Autodesk Fusion 360 part; units mm, degrees
sketch "Sketch1" plane through (0, 0, 0) normal (0, 1, 0) x (1, 0, 0)
  circle A0 centre (0, 0) radius 45
  circle A1 centre (0, 0) radius 2.95
  line L0 (-1.9653, 2.2) -> (1.9653, 2.2)
  circle A2 centre (0, 0) radius 35
  circle A3 centre (0, 0) radius 10
  line L1 (-3.25, 34.8488) -> (-3.25, 9.4571)
  line L2 (3.25, 34.8488) -> (3.25, 9.4571)
  line L3 (-34.1475, 7.6779) -> (-9.9986, -0.1685)
  line L4 (-32.1389, 13.8598) -> (-7.99, 6.0134)
  line L5 (-17.8543, -30.1036) -> (-2.9295, -9.5613)
  line L6 (-23.1129, -26.283) -> (-8.1881, -5.7407)
  line L7 (23.1129, -26.283) -> (8.1881, -5.7407)
  line L8 (17.8543, -30.1036) -> (2.9295, -9.5613)
  line L9 (32.1389, 13.8598) -> (7.99, 6.0134)
  line L10 (34.1475, 7.6779) -> (9.9986, -0.1685)
  line L11 (-0.5, -2.9073) -> (-0.5, -9.9875)
  line L12 (0.5, -2.9073) -> (0.5, -9.9875)
  circle A4 centre (0, 0) radius 42
  dimension "d1" = 90
  dimension "d2" = 5.9
  dimension "d3" = 2.2
  dimension "d4" = 70
  dimension "d5" = 20
  dimension "d6" = 6.5
  dimension "d8" = 360
  dimension "d9" = 1
  dimension "d10" = 84
  dimension "d25" = 25.3916
  dimension "d26" = 20
extrude "Extrude1" add sketch "Sketch1" along normal mid plane 5 contours A0
extrude "Extrude2" add sketch "Sketch1" along normal mid plane 8 contours A4
extrude "Extrude6" add sketch "Sketch1" along normal mid plane 8 contours A1 L0 | A1 A3 L11 L12 | A2 A3 L7 L8 | A2 A3 L5 L6 | A2 A3 L9 L10 | A2 A3 L3 L4 | A2 A3 L1 L2 picked at (-0.7573, 0.4402) picked at (5.7516, 5.0158)
extrude "Extrude7" add sketch "Sketch1" along normal blind 4 contours A1 L0 | A1 A3 L11 L12 picked at (-0.7573, 0.4402) picked at (5.7516, 5.0158)
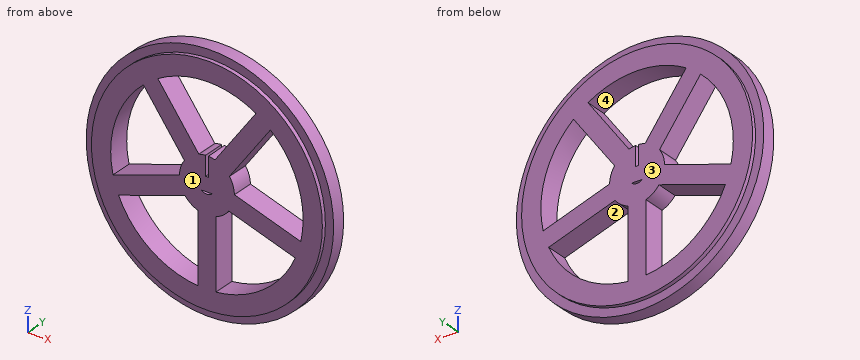
The model under review builds one solid part; all positions refer to its coordinate system, in mm. Face numbers are marked on the shaded views. A direction names the side the tool comes from. Round coordinates to 2 decimals unless told otherwise and drop trailing zeros. Loops run counter-clockwise (first coordinate to the right, second up) from the corner with the lowest first, then second, coordinate; pieces in that order, holes last. Notation, with made-up numbers: M 33,-9.75 L 87,-9.75 A18 cw 87,-3.75 Z; hole C 52.25,29.25 d4. An arc over 180 degrees is marked long. Answer as a JSON object with one key per item and string values.
(1) Tool access review of the marked faces 3 and 4: name each direction out of +Z, -Z, +X, -X, +Y, -Y from which nothing blocks a thin tool from reaching the whole face with its end or side.
Resolved:
{"face 3": "+Z, -Z, +X, -X, +Y", "face 4": "+Y, -Y"}
(2) Take a section at B-B on z = -4. Give the boundary of the cut face in (x, y).
Resolved:
{"outline": "M -44.82,-2.5 L -41.81,-2.5 L -41.81,-4 L -34.77,-4 L -34.77,4 L -41.81,4 L -41.81,2.5 L -44.82,2.5 Z; M -22.83,-4 L 22.83,-4 L 22.83,4 L -22.83,4 Z; M 34.77,-4 L 41.81,-4 L 41.81,-2.5 L 44.82,-2.5 L 44.82,2.5 L 41.81,2.5 L 41.81,4 L 34.77,4 Z"}
(3) Take a section at A-A on x = -12.5. Give the boundary of the cut face in (y, z).
Resolved:
{"outline": "M -4,-40.1 L -2.5,-40.1 L -2.5,-43.23 L 2.5,-43.23 L 2.5,-40.1 L 4,-40.1 L 4,-32.69 L -4,-32.69 Z; M -4,-7.48 L 4,-7.48 L 4,-0.64 L -4,-0.64 Z; M -4,11.68 L 4,11.68 L 4,22.73 L -4,22.73 Z; M -4,32.69 L 4,32.69 L 4,40.1 L 2.5,40.1 L 2.5,43.23 L -2.5,43.23 L -2.5,40.1 L -4,40.1 Z"}
(4) Take a section at D-D on y = 0.25. Give the boundary of the cut face in (x, z), and give its area (3 significant figures).
Resolved:
{"outline": "C 0,0 d90; hole M -34.15,-7.68 L -10,0.17 A10 cw -8.19,5.74 L -23.11,26.28 A35 ccw Z; hole M -32.14,-13.86 A35 ccw -3.25,-34.85 L -3.25,-9.46 A10 cw -7.99,-6.01 Z; hole M -17.85,30.1 L -2.93,9.56 A10 cw -0.5,9.99 L -0.5,2.91 A2.95 cw 0.5,2.91 L 0.5,9.99 A10 cw 2.93,9.56 L 17.85,30.1 A35 ccw Z; hole M -1.97,-2.2 A2.95 ccw 1.97,-2.2 Z; hole M 3.25,-34.85 A35 ccw 32.14,-13.86 L 7.99,-6.01 A10 cw 3.25,-9.46 Z; hole M 8.19,5.74 A10 cw 10,0.17 L 34.15,-7.68 A35 ccw 23.11,26.28 Z", "area": "3,640 mm²"}
(5) To check wall thickness, follow line 1 along X through (y, z) = (1.75, -26); line 2 along Z through (x, y) = (1.5, -1) (3 decimals); line 3 along Z through (x, y) = (-9, -2). State the ranges of each line that lie inside material, in increasing order.
Resolved:
{"line 1": "-36.73 to -23.43, -3.25 to 3.25, 23.43 to 36.73", "line 2": "-44.975 to -2.54, -2.2 to 9.887, 34.968 to 44.975", "line 3": "-44.09 to -33.82, -6.34 to 4.36, 6.86 to 17.92, 33.82 to 44.09"}
(6) Clearance check with flat-ended pins moving along their axes: P1, Ø1.5, axis at y = -1, z = -0.5, coming from the -X side; P2, Ø2.5, axis at y = -1.5, z = -27, coming from the +X side; P3, Ø4, axis at y = 1, z = -21, coming from the -X side; P4, Ø2, axis at x = 1, y = 0.5, coming from the -Z side. State where each tip first meets the part, or that it passes through.
Resolved:
{"P1": "x = -45", "P2": "x = 36.9", "P3": "x = -40.79", "P4": "z = -45"}
(7) Take a section at C-C on x = 20. Give the boundary of the cut face in (y, z), and give its area (3 significant figures).
Resolved:
{"outline": "M -4,-36.93 L -2.5,-36.93 L -2.5,-40.31 L 2.5,-40.31 L 2.5,-36.93 L 4,-36.93 L 4,-28.72 L -4,-28.72 Z; M -4,-9.92 L 4,-9.92 L 4,-3.08 L -4,-3.08 Z; M -4,22 L 4,22 L 4,36.93 L 2.5,36.93 L 2.5,40.31 L -2.5,40.31 L -2.5,36.93 L -4,36.93 Z", "area": "274 mm²"}
(8) Draft analysis for pull direction X (two halves, no side actions). For the marked faces 1 and 2, state which applies: released by +X, released by -X, zero draft, split by the parting line, or undercut.
Resolved:
{"face 1": "zero draft", "face 2": "undercut"}
